Input: part model. Units: mm. Frame: model coordinates. A direction names the side the tool comes from. Round coordinates to 2 decimals unless told otherwise and drop trailing zeros. Order: outer loops, then holes, each group sorted by start corner. A loop starts at its lowest first (then second) coordinate and runs counter-clockwise, first axis right, second up. Notation, with made-up numbers: (51, -2.5) -> (56, -2.5) arc R14 ccw to (56, 12.5) -> close; hole circle Ø4 at (53.5, -9.75). An arc over 180 degrees is marked (long way). Answer as CSV lines item,"result". Start each with the question number.
1) Mould query, pull axis Y, two halves, no side actions, for faces 6 (the face through (-1.463, -33, 2)), 7 (the face through (27, -28, -28)), 8 (the face through (21.094, 13, -10)). Classes: +Y half, -Y half, draft (parallel to the pull), parting line (faces both ways), or undercut.
2) Section query C-C, the plane y = 4.5. Output: boundary loops of the cut face in (x, z).
3) Section query B-B, the plane z = -66. Output: boundary loops of the cut face in (x, y).
4) Section query D-D, the plane x = 19.5. Output: boundary loops of the cut face in (y, z).
5) Access query for faces 1 (the face through (28.094, 20, -10)), 2 (the face through (16, 15, -15)), 3 (the face through (15.769, 24.957, -10.651)), 4 (the face through (22, 5, 0)), 5 (the face through (16, -33, -17)). Directions: +Z, -Z, +X, -X, +Y, -Y. A direction counts if a zero-diameter tool reaches every point of the face in a straight line with its end or side. Return the directions, or none.
6) First-contact query: P1, Ø5.5, axis at y = -32.5, z = 1.5, coming from the +X side; P2, Ø3, axis at y = -12, z = -27.5, coming from the +X side; P3, Ø3, axis at x = 33, z = -41.5, coming from the +Y side. Flat tips, straight axial feed; report the tip coordinate or a pass-through.
7) Section query A-A, the plane x = 43. Output: boundary loops of the cut face in (y, z), and give its area (3 significant figures).
8) Line query: L1, parallel to Y at x = 26, z = -61; L2, parallel to X at y = -33.75, z = -60; L3, parallel to Z at x = 16.5, y = 3.5. Output: solid intervals per line, ascending.
```python
from build123d import *

# Parameters (mm, degrees)
SKETCH1_R                = 13
SKETCH1_R_2              = 7
BOSS_EXTRUDE2_DEPTH      = 10
SKETCH2_R                = 10
BOSS_EXTRUDE3_DEPTH      = 28
SKETCH3_R                = 10
SKETCH3_R_2              = 13
SKETCH3_R_3              = 7
BOSS_EXTRUDE4_DEPTH      = 10
FILLET2_R                = 10
CUT_EXTRUDE1_DEPTH       = 17
BOSS_EXTRUDE5_DEPTH      = 29
BOSS_EXTRUDE5_DEPTH_BACK = 5
SKETCH5_R                = 5
FILLET3_R                = 10
SKETCH6_R                = 10
BOSS_EXTRUDE6_DEPTH      = 10
SKETCH7_W                = 10
SKETCH7_H                = 10
BOSS_EXTRUDE7_DEPTH      = 10
BOSS_EXTRUDE8_DEPTH      = 8
BOSS_EXTRUDE8_DEPTH_BACK = 17
SKETCH8_R                = 5


with BuildPart() as part:
    # Sketch1 → Boss-Extrude2 (new body)
    # profile 1 of 2: a face of its own
    with BuildSketch(Plane(origin=(0, 0, 0), x_dir=(1, 0, 0), z_dir=(0, 1, 0))):
        with BuildLine():
            ThreePointArc((29.247640438, 60), (16.247640438, 47), (3.247640438, 60))
            Line((3.247640438, 60), (-5.462946679, 0))
            Line((-5.462946679, 0), (52.203983694, 0))
            Line((52.203983694, 0), (29.247640438, 60))
        make_face()
    # profile 2 of 2: a face of its own
    with BuildSketch(Plane(origin=(0, 0, 0), x_dir=(1, 0, 0), z_dir=(0, 1, 0))):
        with Locations((16.247640438, 60)):
            Circle(SKETCH1_R)
        with Locations(Location((16.247640438, 60, 0), (0, 0, 270))):
            Circle(SKETCH1_R_2, mode=Mode.SUBTRACT)
    extrude(amount=BOSS_EXTRUDE2_DEPTH)

    # Sketch2 → Boss-Extrude3 (add)
    with BuildSketch(Plane.XZ):
        with Locations(Location((16.05250876, -30, 0), (0, 0, 90))):
            Circle(SKETCH2_R)
    extrude(amount=BOSS_EXTRUDE3_DEPTH)

    # Fillet2
    fillet2_edges = [part.edges().sort_by_distance(p)[0] for p in [
        (52.203983694, 5, 0),
        (-5.462946679, 5, 0),
    ]]
    fillet(fillet2_edges, radius=FILLET2_R)



with BuildPart() as body_2:
    # Sketch3 → Boss-Extrude4 (new body)
    # profile 1 of 2: a face of its own
    with BuildSketch(Plane.XZ.offset(28)):
        with BuildLine():
            Line((-5.462946679, 0), (3.247640438, -60))
            ThreePointArc((3.247640438, -60), (16.247640438, -47), (29.247640438, -60))
            Line((29.247640438, -60), (52.203983694, 0))
            Line((52.203983694, 0), (-5.462946679, 0))
        make_face()
        with Locations(Location((16.05250876, -30, 0), (0, 0, 90))):
            Circle(SKETCH3_R, mode=Mode.SUBTRACT)
    # profile 2 of 2: a face of its own
    with BuildSketch(Plane.XZ.offset(28)):
        with Locations((16.247640438, -60)):
            Circle(SKETCH3_R_2)
        with Locations(Location((16.247640438, -60, 0), (0, 0, 90))):
            Circle(SKETCH3_R_3, mode=Mode.SUBTRACT)
    extrude(amount=BOSS_EXTRUDE4_DEPTH)

    # Sketch4 → Cut-Extrude1 (cut)
    with BuildSketch(Plane.XY):
        Polygon((4.537053321, -33), (4.537053321, -38), (27.537053321, -38), (27.537053321, -28), (4.537053321, -28), align=None)
    extrude(amount=-CUT_EXTRUDE1_DEPTH, mode=Mode.SUBTRACT)

    # Sketch5 → Boss-Extrude5 (add, two sides: drawn at the far end of the back side and taken through both)
    with BuildSketch(Plane.ZY.offset(-27.537053321).offset(-BOSS_EXTRUDE5_DEPTH_BACK)):
        with Locations(Location((0, -33, 0), (0, 0, 270))):
            Circle(SKETCH5_R)
    extrude(amount=BOSS_EXTRUDE5_DEPTH + BOSS_EXTRUDE5_DEPTH_BACK)

    # Fillet3
    # the kernel refuses this fillet: 10 mm, written as the material it takes off along each edge
    with BuildSketch(Plane(origin=(-5.462946679, -6.641526704, 0), x_dir=(0.14367033386913813, 0, -0.989625603531927), z_dir=(0, -1, 0))) as fillet3_piece_1:
        with BuildLine():
            CenterArc((8.543389319, 10), FILLET3_R, 217.167683939, 52.832316061)
            Line((0.574681335, 3.958502414), (0.415307176, 3.837672462))
            ThreePointArc((0.415307176, 3.837672462), (0.089415547, 2.007985274), (-0.197925121, 0.028734067))
            Line((-0.197925121, 0.028734067), (0, -0.2))
            Line((0, -0.2), (8.543389319, -0.2))
            Line((8.543389319, -0.2), (8.543389319, 0))
        make_face()
    extrude(amount=52.716946593, mode=Mode.SUBTRACT)
    with BuildSketch(Plane(origin=(52.203983694, 8.33251049, 0), x_dir=(-0.35734343452809125, 0, -0.9339730562493052), z_dir=(0, -1, 0))) as fillet3_piece_2:
        with BuildLine():
            CenterArc((FILLET3_R * 1.45330041958, -FILLET3_R), FILLET3_R, 90, 110.9371366)
            Line((FILLET3_R * 0.519327363336, -FILLET3_R * 1.35734343453), (FILLET3_R * 0.500647902211, -FILLET3_R * 1.36449030322))
            Line((FILLET3_R * 0.500647902211, -FILLET3_R * 1.36449030322), (-FILLET3_R * 0.0290660083917, FILLET3_R * 0.02))
            Line((-FILLET3_R * 0.0290660083917, FILLET3_R * 0.02), (FILLET3_R * 1.45330041958, FILLET3_R * 0.02))
            Line((FILLET3_R * 1.45330041958, FILLET3_R * 0.02), (FILLET3_R * 1.45330041958, 0))
        make_face()
    extrude(amount=82.665020979, mode=Mode.SUBTRACT)


with BuildPart() as part_1:
    add(part.part)

    add(body_2.part)  # Boss-Extrude6 merges body 2
    # Sketch6 → Boss-Extrude6 (add)
    with BuildSketch(Plane.XZ.offset(28)):
        with Locations(Location((16.05250876, -30, 0), (0, 0, 90))):
            Circle(SKETCH6_R)
    extrude(amount=BOSS_EXTRUDE6_DEPTH)

    # Sketch7 → Boss-Extrude7 (add)
    with BuildSketch(Plane(origin=(0, 10, 0), x_dir=(1, 0, 0), z_dir=(0, 1, 0))):
        with Locations((16.093649369, 10)):
            Rectangle(SKETCH7_W, SKETCH7_H)
    extrude(amount=BOSS_EXTRUDE7_DEPTH)

    # Sketch8 → Boss-Extrude8 (add, two sides: drawn at the far end of the back side and taken through both)
    with BuildSketch(Plane.ZY.offset(-11.093649369).offset(-BOSS_EXTRUDE8_DEPTH_BACK)):
        with Locations((-10, 20)):
            Circle(SKETCH8_R)
    extrude(amount=BOSS_EXTRUDE8_DEPTH + BOSS_EXTRUDE8_DEPTH_BACK)


solid = part_1.part
```
Findings:
1,face 6,"draft"
1,face 7,"undercut"
1,face 8,"undercut"
2,outline,"(-3.8, -11.44) -> (3.25, -60) arc R13 ccw to (29.25, -60) -> (47.01, -13.57) arc R10 ccw to (37.67, 0) -> (6.09, 0) arc R10 ccw to start; hole circle Ø14 at (16.25, -60)"
3,outline,"(4.72, -38) -> (12.64, -38) -> (12.64, -28) -> (4.72, -28) -> close; (4.72, 0) -> (12.64, 0) -> (12.64, 10) -> (4.72, 10) -> close; (19.85, -38) -> (27.78, -38) -> (27.78, -28) -> (19.85, -28) -> close; (19.85, 0) -> (27.78, 0) -> (27.78, 10) -> (19.85, 10) -> close"
4,outline,"(-38, -72.59) -> (-28, -72.59) -> (-28, -66.2) -> (-38, -66.2) -> close; (-38, -53.8) -> (-28, -53.8) -> (-28, -39.39) -> (0, -39.39) -> (0, -53.8) -> (10, -53.8) -> (10, -15) -> (20, -15) arc R5 ccw to (20, -5) -> (10, -5) -> (10, 0) -> (0, 0) -> (0, -20.61) -> (-28, -20.61) -> (-28, -17) -> (-38, -17) -> close; circle Ø10 at (-33, 0); (0, -72.59) -> (10, -72.59) -> (10, -66.2) -> (0, -66.2) -> close"
5,face 1,"+Z, -Z, +X, +Y"
5,face 2,"-Z, +X, -X, +Y"
5,face 3,"none"
5,face 4,"+Z, +X, -X, +Y"
5,face 5,"-Y"
6,P1,"stops at x = 42.51"
6,P2,"stops at x = 26"
6,P3,"stops at y = 10"
7,outline,"(-38, -24.06) -> (-28, -24.06) -> (-28, -1.54) -> (-38, -1.54) -> close; (0, -24.06) -> (10, -24.06) -> (10, -1.54) -> (0, -1.54) -> close"
7,area,"450 mm^2"
8,L1,"y = -38 to -28, 0 to 10"
8,L2,"x = 3.25 to 9.25, 23.25 to 29.25"
8,L3,"z = -73 to -67, -53 to 0"
